Autodesk Inventor part; units mm, degrees
ref_plane "Work Plane1" through (0, 0, 10) normal (0, 0, 1) x (1, 0, 0)
ref_plane "YZ Plane" through (0, 0, 0) normal (1, 0, 0) x (0, 1, 0)
ref_plane "XZ Plane" through (0, 0, 0) normal (0, 1, 0) x (-1, 0, 0)
ref_plane "Work Plane1" through (0, 0, 10) normal (0, 0, 1) x (1, 0, 0)
sketch "Sketch1" plane through (0, 0, 10) normal (0, 0, 1) x (1, 0, 0)
  line L0 (-4.0299, -0.3538) -> (-2.2322, 1.4439) construction
  arc A0 (-1.4439, 2.2322) -> (-2.2322, 1.4439) centre (-0.9299, 0.9299) ccw construction
  line L1 (-1.4439, 2.2322) -> (0.3538, 4.0299) construction
  line L2 (-37.8299, 42.8299) -> (-37.8299, 37.8299) construction
  line L3 (-37.8299, 37.8299) -> (-42.9208, 37.8299) construction
  line L4 (-37.8299, 42.2137) -> (-37.8299, 45.8299) construction
  line L5 (-37.8299, 45.8299) -> (-4.0299, 45.8299) construction
  line L6 (-4.0299, 45.8299) -> (-4.0299, 42.2137) construction
  line L7 (-4.0299, 4.0299) -> (0.3538, 4.0299)
  circle A1 centre (-20.9299, 20.9299) radius 17.5
  line L8 (-20.9299, 58.9723) -> (17.1124, 20.9299) construction
  line L9 (17.1124, 20.9299) -> (-20.9299, -17.1124) construction
  line L10 (-20.9299, -17.1124) -> (-58.9723, 20.9299) construction
  line L11 (-58.9723, 20.9299) -> (-20.9299, 58.9723) construction
  line L12 (-20.9299, 58.9723) -> (-20.9299, -17.1124) construction
  line L13 (17.1124, 20.9299) -> (-58.9723, 20.9299) construction
  line L14 (-20.9299, 58.9723) -> (32.8701, 58.9723) construction
  line L15 (-43.4299, 43.4299) -> (1.5701, 43.4299) construction
  line L16 (1.5701, 43.4299) -> (1.5701, -1.5701) construction
  line L17 (1.5701, -1.5701) -> (-43.4299, -1.5701) construction
  line L18 (-43.4299, -1.5701) -> (-43.4299, 43.4299) construction
  line L19 (-43.4299, 43.4299) -> (1.5701, -1.5701) construction
  line L20 (1.5701, 43.4299) -> (-43.4299, -1.5701) construction
  line L21 (-43.4299, 5.3876) -> (-43.4299, 36.4723)
  line L22 (-43.4299, 36.4723) -> (-36.4723, 43.4299)
  line L23 (-36.4723, 43.4299) -> (-5.3876, 43.4299)
  line L24 (-5.3876, 43.4299) -> (1.5701, 36.4723)
  line L25 (1.5701, 36.4723) -> (1.5701, 5.3876)
  line L26 (1.5701, 5.3876) -> (-5.3876, -1.5701)
  line L27 (-5.3876, -1.5701) -> (-36.4723, -1.5701)
  line L28 (-36.4723, -1.5701) -> (-43.4299, 5.3876)
  line L29 (-4.0299, 42.2137) -> (-37.8299, 42.2137)
  line L30 (-4.0299, -0.3538) -> (-4.0299, 4.0299)
  circle A2 centre (-20.9299, 20.9299) radius 1.5
  line L31 (-10.9299, 10.9299) -> (-30.9299, 10.9299) construction
  line L32 (-30.9299, 10.9299) -> (-30.9299, 30.9299) construction
  line L33 (-30.9299, 30.9299) -> (-10.9299, 30.9299) construction
  line L34 (-10.9299, 30.9299) -> (-10.9299, 10.9299) construction
  line L35 (-10.9299, 10.9299) -> (-30.9299, 30.9299) construction
  line L36 (-30.9299, 10.9299) -> (-10.9299, 30.9299) construction
  circle A3 centre (-30.9299, 30.9299) radius 1.4
  circle A4 centre (-30.9299, 10.9299) radius 1.4
  circle A5 centre (-10.9299, 10.9299) radius 1.4
  line L37 (-45.8299, 37.8299) -> (-42.0723, 37.8299) construction
  line L38 (-42.1723, 37.7299) -> (-45.8299, 37.7299)
  line L39 (-45.8299, 37.7299) -> (-45.8299, 4.1299)
  line L40 (-45.8299, 4.1299) -> (-42.1723, 4.1299)
  line L41 (-42.1723, 4.1299) -> (-42.1723, 37.7299)
  line L42 (-45.8299, 4.0299) -> (-42.0723, 4.0299) construction
  line L43 (-45.8299, 37.8299) -> (-42.0723, 37.8299)
  line L44 (-37.7299, 45.8299) -> (-4.1299, 45.8299)
  line L45 (-4.1299, 45.8299) -> (-4.1299, 42.1723)
  line L46 (-4.1299, 42.1723) -> (-37.7299, 42.1723)
  line L47 (-37.7299, 42.1723) -> (-37.7299, 45.8299)
  line L48 (0.4701, 37.8299) -> (0.4701, 4.0299) construction
  line L49 (0.4701, 4.0299) -> (3.9701, 4.0299) construction
  line L50 (3.9701, 37.8299) -> (3.9701, 4.0299) construction
  line L51 (0.4701, 37.8299) -> (3.9701, 37.8299) construction
  line L52 (-45.8299, -3.9701) -> (-4.0299, -3.9701) construction
  line L53 (0.3124, 37.7299) -> (3.9701, 37.7299)
  line L54 (3.9701, 37.7299) -> (3.9701, 4.1299)
  line L55 (3.9701, 4.1299) -> (0.3124, 4.1299)
  line L56 (0.3124, 4.1299) -> (0.3124, 37.7299)
  line L57 (-4.1713, -0.3538) -> (-37.7299, -0.3538)
  line L58 (-37.7299, -0.3538) -> (-37.7299, -3.9701)
  line L59 (-37.7299, -3.9701) -> (-4.1713, -3.9701)
  line L60 (-4.1713, -3.9701) -> (-4.1713, -0.3538)
  point P0 (-37.8299, 4.0299)
  dimension "d18" = 53.8
  dimension "d19" = 45
  dimension "d20" = 53.8
  dimension "d21" = 45
  dimension "d22" = 45
  dimension "d30" = 20
  dimension "d31" = 20
  dimension "d32" = 2.8
  dimension "d33" = 2.8
  dimension "d34" = 2.8
  dimension "d35" = 3
  dimension "d36" = 0.1
  dimension "d37" = 0.1
  dimension "d38" = 0.1
  dimension "d39" = 0.1
extrude "Extrusion1" add sketch "Sketch1" along normal blind 10 contours L30 L26 L57 L28 L41 L22 L46 L24 L56 L7 | L7 L26 L30 | L56 L24 L25 L26 | L26 L25 L24 L53 L54 L55 | L60 L59 L58 L57 L28 L27 L26 | L26 L27 L28 L57 | L46 L22 L29 L24 | L24 L29 L45 | L40 L39 L38 L22 L21 L28 | L28 L21 L22 L41 | L29 L22 L23 L24 | L24 L23 L22 L29 L47 L44 L45 | L47 L29 L22 | A1 | A2 | A3 | A4 | A5
sketch "Skizze4" plane through (0, 0, 20) normal (0, 0, 1) x (1, 0, 0)
  line L0 (-37.7299, 42.1723) -> (-42.1723, 37.7299)
  line L1 (-42.1723, 37.7299) -> (-45.8299, 37.7299)
  line L2 (-45.8299, 37.7299) -> (-45.8299, 4.1299) construction
  line L3 (-45.8299, 4.1299) -> (-42.1723, 4.1299)
  line L4 (-42.1723, 4.1299) -> (-37.6885, -0.3538)
  line L5 (-37.6885, -0.3538) -> (-37.7299, -0.3538)
  line L6 (-37.7299, -0.3538) -> (-37.7299, -3.9701)
  line L7 (-37.7299, -3.9701) -> (-4.1713, -3.9701) construction
  line L8 (-4.1713, -3.9701) -> (-4.1713, -0.3538)
  line L9 (-4.1713, -0.3538) -> (0.3124, 4.1299)
  line L10 (0.3124, 4.1299) -> (3.9701, 4.1299)
  line L11 (3.9701, 4.1299) -> (3.9701, 37.7299) construction
  line L12 (3.9701, 37.7299) -> (0.3124, 37.7299)
  line L13 (0.3124, 37.7299) -> (-4.1299, 42.1723)
  line L14 (-4.1299, 42.1723) -> (-4.1299, 45.8299)
  line L15 (-4.1299, 45.8299) -> (-37.7299, 45.8299) construction
  line L16 (-37.7299, 45.8299) -> (-37.7299, 42.1723)
  line L17 (-37.9299, 46.0299) -> (-3.9299, 46.0299) construction
  line L18 (-3.9299, 46.0299) -> (-3.9299, 42.2551)
  line L19 (-3.9299, 42.2551) -> (0.3953, 37.9299)
  line L20 (0.3953, 37.9299) -> (4.1701, 37.9299)
  line L21 (4.1701, 37.9299) -> (4.1701, 3.9299) construction
  line L22 (4.1701, 3.9299) -> (0.3953, 3.9299)
  line L23 (0.3953, 3.9299) -> (-3.9713, -0.4367)
  line L24 (-3.9713, -0.4367) -> (-3.9713, -4.1701)
  line L25 (-3.9713, -4.1701) -> (-37.9299, -4.1701) construction
  line L26 (-37.9299, -4.1701) -> (-37.9299, -0.3953)
  line L27 (-37.9299, -0.3953) -> (-42.2551, 3.9299)
  line L28 (-42.2551, 3.9299) -> (-46.0299, 3.9299)
  line L29 (-46.0299, 3.9299) -> (-46.0299, 37.9299) construction
  line L30 (-46.0299, 37.9299) -> (-42.2551, 37.9299)
  line L31 (-42.2551, 37.9299) -> (-37.9299, 42.2551)
  line L32 (-37.9299, 42.2551) -> (-37.9299, 46.0299)
  line L33 (-45.8299, 37.7299) -> (-45.8299, 37.9299)
  line L34 (-4.1299, 45.8299) -> (-37.7299, 45.8299)
  line L35 (-37.7299, 45.8299) -> (-37.9299, 45.8299)
  line L36 (-4.1299, 45.8299) -> (-3.9299, 45.8299)
  line L37 (3.9701, 37.7299) -> (3.9701, 37.9299)
  line L38 (3.9701, 4.1299) -> (3.9701, 37.7299)
  line L39 (3.9701, 4.1299) -> (3.9701, 3.9299)
  line L40 (-4.1713, -3.9701) -> (-3.9713, -3.9701)
  line L41 (-37.7299, -3.9701) -> (-37.9299, -3.9701)
  line L42 (-45.8299, 4.1299) -> (-45.8299, 3.9299)
  point P0 (0, 0)
  dimension "d40" = 0.2
extrude "IM_offset" add sketch "Skizze4" against normal up to surface (10 mm away)
ref_plane "Work Plane5" through (-37.9299, 20.9299, 10) normal (0, -1, 0) x (1, 0, 0)
ref_plane "Work Plane6" through (-20.9299, 3.9299, 10) normal (1, 0, 0) x (0, 0, -1)
sketch "Sketch24" plane through (0, 0, 10) normal (0, 0, -1) x (-1, 0, 0)
  line L0 (6.4299, 6.4299) -> (35.4299, 6.4299) construction
  line L1 (35.4299, 6.4299) -> (35.4299, 35.4299) construction
  line L2 (35.4299, 35.4299) -> (6.4299, 35.4299) construction
  line L3 (6.4299, 35.4299) -> (6.4299, 6.4299) construction
  line L4 (6.4299, 6.4299) -> (35.4299, 35.4299) construction
  line L5 (35.4299, 6.4299) -> (6.4299, 35.4299) construction
  point P0 (0, 0)
  point P1 (20.9299, 20.9299)
  dimension "d143" = 29
  dimension "d144" = 29
hole "Hole1" at (-20.9299, 20.9299, 10) at (-6.4299, 6.4299, 10) at (-35.4299, 6.4299, 10) at (-35.4299, 35.4299, 10) at (-6.4299, 35.4299, 10) direction (0, 0, 1) diameter 4.1 end through all
sketch "Skizze28" plane through (0, 0, 10) normal (0, 0, -1) x (-1, 0, 0)
  circle A0 centre (25.9299, 6.9299) radius 3
  circle A1 centre (6.9299, 25.9299) radius 3
  line L0 (9.9299, 4.9299) -> (1.9299, 4.9299)
  line L1 (4.9299, 1.9299) -> (1.9299, 4.9299)
  line L2 (36.9299, 1.9299) -> (4.9299, 1.9299)
  line L3 (39.9299, 4.9299) -> (36.9299, 1.9299)
  line L4 (39.9299, 36.9299) -> (39.9299, 4.9299)
  line L5 (36.9299, 39.9299) -> (39.9299, 36.9299)
  line L6 (4.9299, 39.9299) -> (36.9299, 39.9299)
  line L7 (1.9299, 36.9299) -> (4.9299, 39.9299)
  line L8 (1.9299, 8.9299) -> (1.9299, 36.9299)
  line L9 (1.9299, 8.9299) -> (9.9299, 8.9299)
  line L10 (9.9299, 8.9299) -> (9.9299, 4.9299)
  circle A2 centre (34.9299, 6.9299) radius 2
  circle A3 centre (6.9299, 25.9299) radius 4.05
  circle A4 centre (25.9299, 6.9299) radius 4.05
  point P0 (0, 0)
  dimension "d173" = 8.1
  dimension "d174" = 8.1
extrude "Extrusion23" cut sketch "Skizze28" against normal blind 9.5 contours A0 | A1 | A3 | A4
chamfer "Fase2" distance 0.5 angle 45 27 edges at (-2.8799, 25.9299, 10) (-35.4299, 4.3799, 10) (-6.4299, 4.3799, 10) (-20.9299, 18.8799, 10) (-35.4299, 33.3799, 10) (-6.4299, 33.3799, 10) (-21.8799, 6.9299, 10) (-45.8299, 20.9299, 10) (-20.9506, -3.9701, 10) (3.9701, 20.9299, 20) (3.9701, 20.9299, 10) (-20.9299, 45.8299, 10) (-44.0425, 37.9299, 20) (-40.0925, 40.0925, 20) (-37.9299, 44.0425, 20) (-20.9299, 45.8299, 20) (-45.8299, 20.9299, 20) (-44.0425, 3.9299, 20) (-20.9506, -3.9701, 20) (-37.9299, -2.1827, 20) (-40.0925, 1.7673, 20) (-3.9713, -2.2034, 20) (-1.788, 1.7466, 20) (2.1827, 3.9299, 20) (2.1827, 37.9299, 20) (-1.7673, 40.0925, 20) (-3.9299, 44.0425, 20)
sketch "Skizze29" plane through (0, 0, 20) normal (0, 0, 1) x (1, 0, 0)
  circle A0 centre (-35.4299, 6.4299) radius 2.55
  circle A1 centre (-25.9299, 6.9299) radius 4.55
  circle A2 centre (-20.9299, 20.9299) radius 2.55
  circle A3 centre (-6.9299, 25.9299) radius 4.55
  circle A4 centre (-6.4299, 35.4299) radius 2.55
  circle A5 centre (-6.4299, 6.4299) radius 2.55
  circle A6 centre (-35.4299, 35.4299) radius 2.55
  line L0 (3.4701, 4.4299) -> (3.4701, 37.4299)
  line L1 (0.1882, 4.4299) -> (3.4701, 4.4299)
  line L2 (-4.4713, -0.2296) -> (0.1882, 4.4299)
  line L3 (-4.4713, -3.4701) -> (-4.4713, -0.2296)
  line L4 (-37.4299, -3.4701) -> (-4.4713, -3.4701)
  line L5 (-37.4299, -0.1882) -> (-37.4299, -3.4701)
  line L6 (-42.048, 4.4299) -> (-37.4299, -0.1882)
  line L7 (-45.3299, 4.4299) -> (-42.048, 4.4299)
  line L8 (-45.3299, 37.4299) -> (-45.3299, 4.4299)
  line L9 (-42.048, 37.4299) -> (-45.3299, 37.4299)
  line L10 (-37.4299, 42.048) -> (-42.048, 37.4299)
  line L11 (-37.4299, 45.3299) -> (-37.4299, 42.048)
  line L12 (-4.4299, 45.3299) -> (-37.4299, 45.3299)
  line L13 (-4.4299, 42.048) -> (-4.4299, 45.3299)
  line L14 (0.1882, 37.4299) -> (-4.4299, 42.048)
  line L15 (3.4701, 37.4299) -> (0.1882, 37.4299)
  point P0 (0, 0)
hole "Bohrung2" at (-6.9299, 25.9299, 20) at (-25.9299, 6.9299, 20) direction (0, 0, -1) diameter 6 end through all
sketch "Sketch30" plane through (3.9701, 3.9299, 19.5) normal (1, 0, 0) x (0, 0, -1)
  line L0 (9.5, 44.7711) -> (7.5, 44.7711)
  line L1 (7.5, 44.7711) -> (7.5, -17.5234)
  line L2 (7.5, -17.5234) -> (9.5, -17.5234)
  line L3 (9.5, -17.5234) -> (9.5, 44.7711)
  line L4 (9.5, 0.5) -> (9.5, 33.5)
  point P0 (19.5, -3.9299)
  dimension "d187" = 2
extrude "Extrusion24" cut sketch "Sketch30" against normal through all
properties part number "20_Cube_Insert_Kinematic_Mirror_90_pro_magnetic"
Design review of the part built by this model. Coordinates are the model's own, in mm. A direction names the side the tool comes from. Round coordinates to 2 decimals unless told otherwise and drop trailing zeros. Order: outer loops, then holes, each group sorted by start corner. A loop starts at its lowest first (then second) coordinate and runs counter-clockwise, first axis right, second up. Notation, with made-up numbers: (58, 67) - (77, 67) arc R10 ccw to (77, 84) - close; hole circle Ø2 at (-27, -22.75). An arc over 180 degrees is marked (long way). Return JSON: item names as keys, results as strings.
Q1. Machinability: for faces 1 (the flat face through (2, 3.93, 16)), 2 (the flat face through (-4, 24, 19.5)), 3 (the flat face through (-44, 3.93, 16)), which of the approach directions +Z, -Z, +X, -X, +Y, -Y give a long, thin tool a straight path to every point of the face, cutting with its end or side? Answer none if there is none.
Computed values:
{"face 1": "+Z, -Z, +X, -Y", "face 2": "-Z", "face 3": "+Z, -Z, -X, -Y"}
Q2. Consider section D-D on z = 13.5. Write out the cut boundary in (x, y), plus the area to 3 significant figures.
Computed values:
{"outline": "(-45.83, 3.93) - (-42.26, 3.93) - (-37.93, -0.4) - (-37.93, -3.97) - (-3.97, -3.97) - (-3.97, -0.44) - (0.4, 3.93) - (3.97, 3.93) - (3.97, 37.93) - (0.4, 37.93) - (-3.93, 42.26) - (-3.93, 45.83) - (-37.93, 45.83) - (-37.93, 42.26) - (-42.26, 37.93) - (-45.83, 37.93) - close; hole circle Ø4.1 at (-35.43, 6.43); hole circle Ø4.1 at (-35.43, 35.43); hole circle Ø8.1 at (-25.93, 6.93); hole circle Ø4.1 at (-20.93, 20.93); hole circle Ø8.1 at (-6.93, 25.93); hole circle Ø4.1 at (-6.43, 6.43); hole circle Ø4.1 at (-6.43, 35.43)", "area": "2,100 mm2"}
Q3. Consider section B-B on y = 27.5. Write out the cut boundary in (x, z).
Computed values:
{"outline": "(-45.83, 12) - (-10.66, 12) - (-10.66, 19.5) - (-9.49, 19.5) - (-9.49, 20) - (-45.33, 20) - (-45.83, 19.5) - close; (-4.37, 19.5) - (-3.2, 19.5) - (-3.2, 12) - (3.97, 12) - (3.97, 19.5) - (3.47, 20) - (-4.37, 20) - close"}
Q4. The part is to be moulded in two halves that separate along Y. For faces 4 (the cylindrical face through (-37.16, 36.53, 16.06)), 5 (the flat face through (-39.88, 1.91, 19.75)), 6 (the cylindrical face through (-6.403, 29.945, 15.698)), 7 (the flat face through (-3.971, -2, 16)), say which applies: pulls with the +Y half, pulls with the -Y half, needs draft (parallel to the pull), parting line crosses it, or undercut.
Computed values:
{"face 4": "undercut", "face 5": "pulls with the -Y half", "face 6": "undercut", "face 7": "needs draft"}
Q5. Consider section A-A on x = -24. Write out the cut boundary in (y, z).
Computed values:
{"outline": "(-3.97, 12) - (3.37, 12) - (3.37, 19.5) - (4.63, 19.5) - (4.63, 20) - (-3.47, 20) - (-3.97, 19.5) - close; (9.23, 19.5) - (10.49, 19.5) - (10.49, 12) - (45.83, 12) - (45.83, 19.5) - (45.33, 20) - (9.23, 20) - close"}
Q6. Consider section C-C on y = 5. Write out the cut boundary in (x, z), plus the area to 3 significant figures.
Computed values:
{"outline": "(-45.83, 12) - (-36.9, 12) - (-36.9, 20) - (-45.33, 20) - (-45.83, 19.5) - close; (-33.96, 12) - (-29.49, 12) - (-29.49, 19.5) - (-28.23, 19.5) - (-28.23, 20) - (-33.96, 20) - close; (-23.63, 19.5) - (-22.37, 19.5) - (-22.37, 12) - (-7.9, 12) - (-7.9, 20) - (-23.63, 20) - close; (-4.96, 12) - (3.97, 12) - (3.97, 19.5) - (3.47, 20) - (-4.96, 20) - close", "area": "295 mm2"}
Q7. For pin 1 Ø4 at (y, z) = (-2, 17) entering from +X; pin 2 Ø4 at (x, z) = (-44, 15) entering from -Y; pin 3 Ø4 at (x, z) = (2.5, 16) entering from -Y, all flat-tipped, find the tip position at first contact; note any pin that passes through.
Computed values:
{"pin 1": "stops at x = -3.53", "pin 2": "stops at y = 3.67", "pin 3": "stops at y = 3.93"}
Q8. Wall thickness on L1, parallel to Y at x = -21, z = 13; L2, parallel to Y at x = -8, z = 18.25; L3, parallel to Y at x = -35, z = 19.25: over which ranges is each line inside the solid? List them lowest first. Write a range as [from, to].
Computed values:
{"L1": "y = [-3.97, 18.88], [22.98, 45.83]", "L2": "y = [-3.97, 5.11], [7.75, 22.02], [29.84, 34.11], [36.75, 45.83]", "L3": "y = [-3.97, 4.43], [8.43, 33.43], [37.43, 45.83]"}
